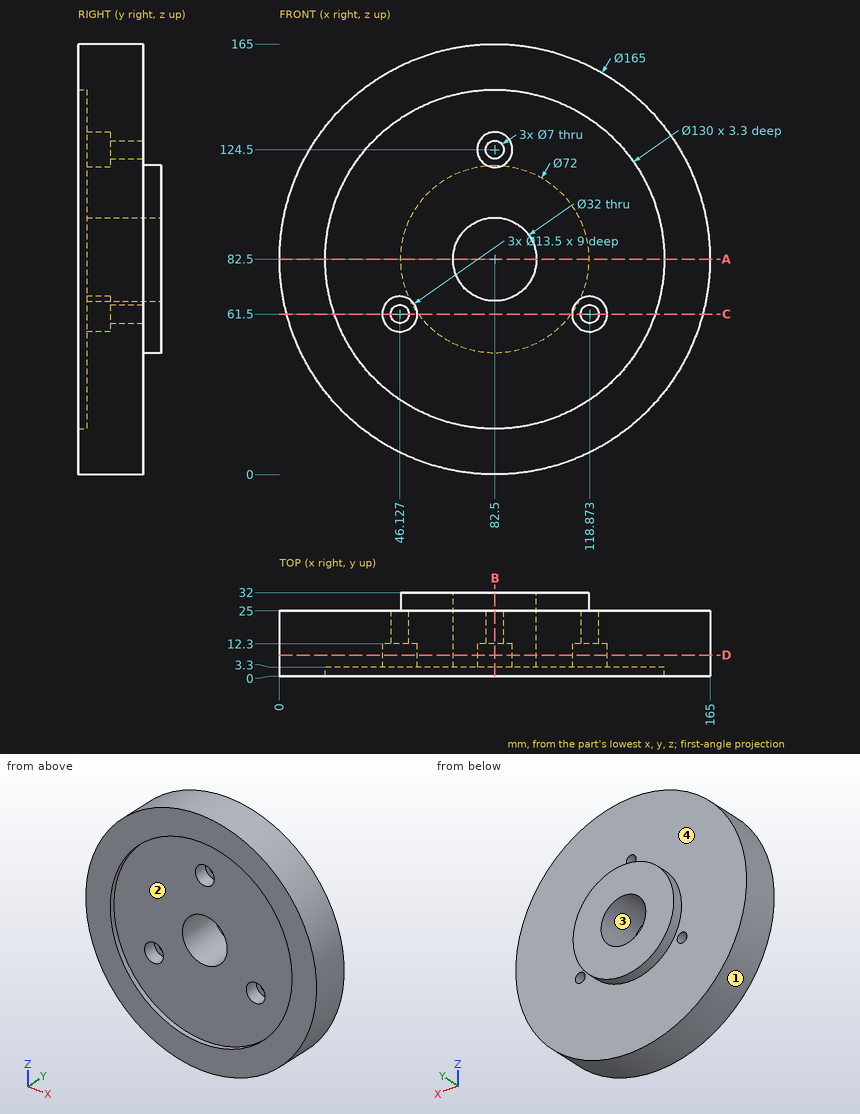
Print and shaded views of the part. All mm, measured from the part's lowest x, y and z. Give positions to 0.01 mm unless a question says otherwise; leave off trailing zeros. Write each loop counter-clockwise with the first axis right and the second up, starting at its lowest first coordinate (ties: lowest second). Pieces come first, ordered by that corner, then holes. Notation, with made-up numbers: (50.25, -13) -> (73.25, -13) arc R16 cw to (73.25, 2) -> close; hole circle Ø5 at (68, 83). An arc over 180 degrees is marked (long way). Write item = value, one per line.
(1) Slice it at D-D, the plane y = 8. Give the cut face in (x, z), then the cut area to 3 significant figures.
Determined:
outline = circle Ø165 at (82.5, 82.5); hole circle Ø13.5 at (46.13, 61.5); hole circle Ø32 at (82.5, 82.5); hole circle Ø13.5 at (82.5, 124.5); hole circle Ø13.5 at (118.87, 61.5)
area = 20,100 mm2
(2) Flat gauge pins, fed straight in: P1, Ø8, axis at x = 142.5, y = 12, coming from the -Z side; P2, Ø2, axis at x = 47.5, z = 41.5, coming from the +Y side; P3, Ø3, axis at y = 4, z = 29, coming from the -X side; P4, Ø1.5, axis at x = 28.5, y = 27, coming from the +Z side. Where does each tip first touch, or does it go through?
Determined:
P1 = 21.92
P2 = 25
P3 = 18.45
P4 = through
(3) Probe line 1 along Z through (x, y) = (82, 14); line 2 along X through (y, z) = (17, 82); line 3 along X through (y, z) = (1.1, 82.5). List the from-to ranges inside material, lowest first.
Determined:
line_1 = 0 to 66.51, 98.49 to 121.04, 127.96 to 165
line_2 = 0 to 66.51, 98.49 to 165
line_3 = 0 to 17.5, 147.5 to 165
(4) Slice it at A-A, the plane z = 82.5. Give the cut face in (x, y), then the cut area to 3 significant figures.
Determined:
outline = (0, 0) -> (17.5, 0) -> (17.5, 3.3) -> (66.5, 3.3) -> (66.5, 32) -> (46.5, 32) -> (46.5, 25) -> (0, 25) -> close; (98.5, 3.3) -> (147.5, 3.3) -> (147.5, 0) -> (165, 0) -> (165, 25) -> (118.5, 25) -> (118.5, 32) -> (98.5, 32) -> close
area = 3,280 mm2
(5) Slice it at B-B, the plane x = 82.5. Give the cut face in (y, z).
Determined:
outline = (0, 0) -> (25, 0) -> (25, 46.5) -> (32, 46.5) -> (32, 66.5) -> (3.3, 66.5) -> (3.3, 17.5) -> (0, 17.5) -> close; (0, 147.5) -> (3.3, 147.5) -> (3.3, 131.25) -> (12.3, 131.25) -> (12.3, 128) -> (25, 128) -> (25, 165) -> (0, 165) -> close; (3.3, 98.5) -> (32, 98.5) -> (32, 118.5) -> (25, 118.5) -> (25, 121) -> (12.3, 121) -> (12.3, 117.75) -> (3.3, 117.75) -> close
(6) Mould opens along Z. For the marked faces 1, 2, 3 and 4 say: released by +Z, released by -Z, zero draft, split by the parting line, or undercut.
Determined:
face_1 = split by the parting line
face_2 = undercut
face_3 = undercut
face_4 = zero draft
(7) Slice it at C-C, the plane z = 61.5. Give the cut face in (x, y).
Determined:
outline = (2.72, 0) -> (20.99, 0) -> (20.99, 3.3) -> (39.38, 3.3) -> (39.38, 12.3) -> (42.63, 12.3) -> (42.63, 25) -> (2.72, 25) -> close; (49.63, 12.3) -> (52.88, 12.3) -> (52.88, 3.3) -> (112.12, 3.3) -> (112.12, 12.3) -> (115.37, 12.3) -> (115.37, 25) -> (111.74, 25) -> (111.74, 32) -> (53.26, 32) -> (53.26, 25) -> (49.63, 25) -> close; (122.37, 12.3) -> (125.62, 12.3) -> (125.62, 3.3) -> (144.01, 3.3) -> (144.01, 0) -> (162.28, 0) -> (162.28, 25) -> (122.37, 25) -> close
